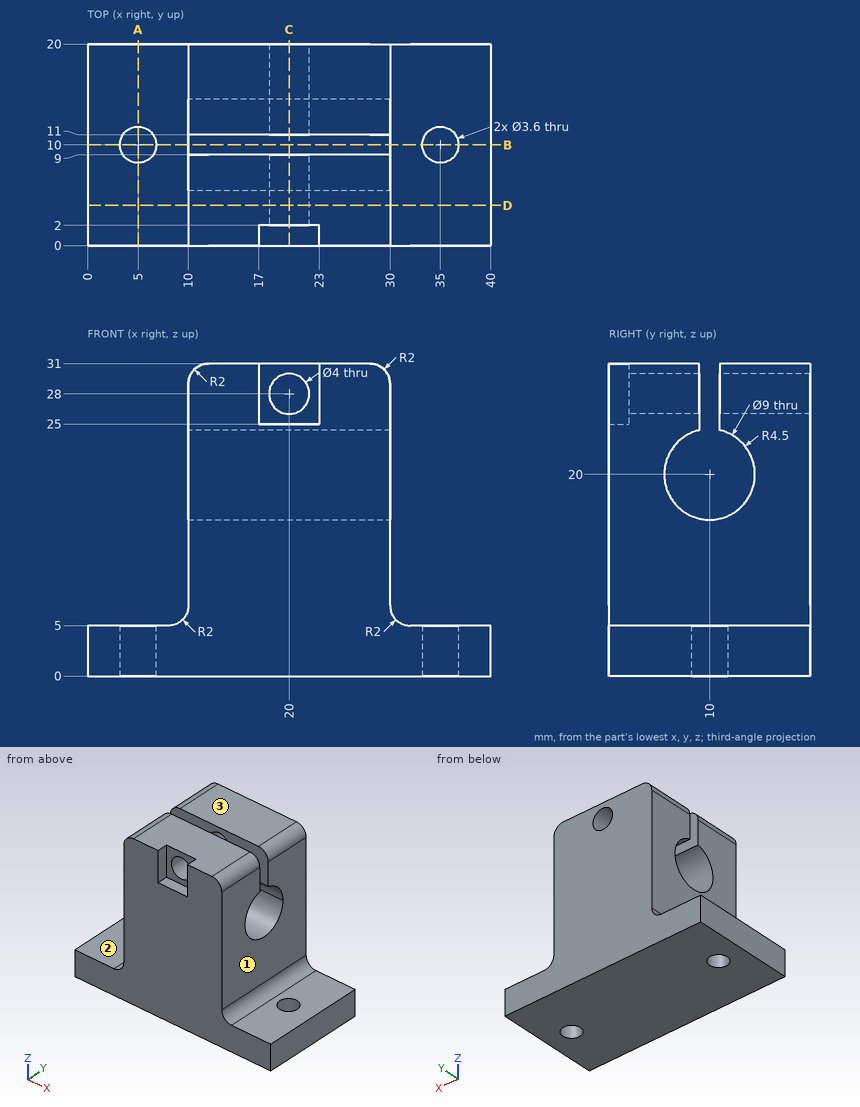
Verification items for this drawing (mm, ordinates from the low corner). A direction names the side the tool comes from. Coordinates: 2 decimals unless noted, no trailing zeros. Loops run counter-clockwise (first coordinate to the right, second up) from the corner with the lowest first, then second, coordinate; pieces in that order, holes last. Notation, with made-up numbers: (3, -32.5) - (43, -32.5) arc R16 cw to (43, -19.5) - close; hole circle Ø11 at (65, 69.25). An arc over 180 degrees is marked (long way). Use one line per item in the form item = value. Start each with the question number.
Item 1: Section check C-C, the plane x = 20. Enter the section's corners in (y, z).
Item 2: Section check D-D, the plane y = 4. Enter the section's corners in (x, z).
Item 3: Gauge pin test, flat ends, axial feed: pin 1 (3.5 mm diameter, centred on x = 16, z = 26.5, fed in from -Y); pin 2 (4 mm diameter, centred on y = 8.5, z = 16.5, fed in from +X); pin 3 (2.5 mm diameter, centred on x = 34.5, y = 6.5, fed in from +Z); pin 4 (1 mm diameter, centred on x = 28, y = 10, fed in from +Z). Record the tip position at first contact, or that the pin passes through.
Item 4: Tool access check on the marked faces 1, 2 and 3. Record the directions out of +Z, -Z, +X, -X, +Y, -Y that give a thin tool (end or side, any length) a straight path to the whole face; none if there is none.
Item 5: Section check B-B, the plane y = 10. Enter the section's corners in (x, z).
Item 6: Thickness scan on probe 1 along X at (y, z) = (10, 2.95); probe 2 along Z at (x, y) = (20, 14); probe 3 along Y at (x, z) = (17.5, 26.5). Record the ranges inside material, lowest first.
Item 7: Section check A-A, the plane x = 5. Enter the section's corners in (y, z), and give its area (3 significant figures).
Computed:
q1.outline = (0, 0) - (20, 0) - (20, 26) - (11, 26) - (11, 24.39) arc R4.5 cw (long way) to (9, 24.39) - (9, 26) - (2, 26) - (2, 25) - (0, 25) - close; (2, 30) - (9, 30) - (9, 31) - (2, 31) - close; (11, 30) - (20, 30) - (20, 31) - (11, 31) - close
q2.outline = (0, 0) - (40, 0) - (40, 5) - (32, 5) arc R2 cw to (30, 7) - (30, 29) arc R2 ccw to (28, 31) - (12, 31) arc R2 ccw to (10, 29) - (10, 7) arc R2 cw to (8, 5) - (0, 5) - close; hole circle Ø4 at (20, 28)
q3.pin_1 = 0
q3.pin_2 = 30
q3.pin_3 = 5
q3.pin_4 = 15.53
q4.face_1 = +Z, +X, +Y, -Y
q4.face_2 = +Z, -X, +Y, -Y
q4.face_3 = +Z, +X, -X, +Y, -Y
q5.outline = (0, 0) - (3.2, 0) - (3.2, 5) - (0, 5) - close; (6.8, 0) - (33.2, 0) - (33.2, 5) - (32, 5) arc R2 cw to (30, 7) - (30, 15.5) - (10, 15.5) - (10, 7) arc R2 cw to (8, 5) - (6.8, 5) - close; (36.8, 0) - (40, 0) - (40, 5) - (36.8, 5) - close
q6.probe_1 = 0 to 3.2, 6.8 to 33.2, 36.8 to 40
q6.probe_2 = 0 to 17.94, 22.06 to 26, 30 to 31
q6.probe_3 = 2 to 9, 11 to 20
q7.outline = (0, 0) - (8.2, 0) - (8.2, 5) - (0, 5) - close; (11.8, 0) - (20, 0) - (20, 5) - (11.8, 5) - close
q7.area = 82.0 mm2
